from build123d import *

# Parameters (mm, degrees)
GAP_DEPTH               = 39.247748954
CUT_EXTRUDE1_DEPTH      = 6.35
CUT_EXTRUDE1_DEPTH_BACK = 6.35
SKETCH3_R               = 4.928370377
SKETCH3_R_2             = 2.3495


with BuildPart() as part:
    # Sketch1 → Base-Revolve (revolve)
    with BuildSketch(Plane.XY, mode=Mode.PRIVATE) as base_revolve_sk:
        Polygon((0, 1.3589), (38.1, 1.3589), (38.1, 2.159), (36.703, 2.3749), (1.397, 2.3749), (0, 2.159), align=None)
    revolve(base_revolve_sk.sketch.rotate(Axis((-9.525, 0, 0), (1, 0, 0)), 90), axis=Axis((-9.525, 0, 0), (1, 0, 0)))

    # Sketch2 → Gap (cut, through all)
    with BuildSketch(Plane(origin=(0, 0, 0), x_dir=(0, -1, 0), z_dir=(-1, 0, 0))):
        with BuildLine():
            Line((0, 0), (0.190059157, 2.414930555))
            ThreePointArc((0.190059157, 2.414930555), (0, 2.422398), (-0.190059157, 2.414930555))
            Line((-0.190059157, 2.414930555), (0, 0))
        make_face()
    extrude(amount=-GAP_DEPTH, mode=Mode.SUBTRACT)

    # Sketch3 → Cut-Extrude1 (cut, two sides: drawn at the far end of the back side and taken through both)
    with BuildSketch(Plane(origin=(17.78, 0, 0), x_dir=(0, 0, -1), z_dir=(1, 0, 0)).offset(-CUT_EXTRUDE1_DEPTH_BACK)):
        Circle(SKETCH3_R)
        Circle(SKETCH3_R_2, mode=Mode.SUBTRACT)
    extrude(amount=CUT_EXTRUDE1_DEPTH + CUT_EXTRUDE1_DEPTH_BACK, mode=Mode.SUBTRACT)


solid = part.part
Source: CAD feature listing. Evaluate the final solid. Frame: model axes, mm. A direction names the side the tool comes from. Coordinates: 2 decimals unless noted, no trailing zeros. Write each loop counter-clockwise with the first axis right and the second up, starting at its lowest first coordinate (ties: lowest second). Pieces come first, ordered by that corner, then holes. Notation, with made-up numbers: M -30,62.5 L 5,62.5 A13 ccw 5,79.5 Z; hole C 59.25,-28 d11. An arc over 180 degrees is marked long. Use a Markdown table: item, result.
1) Section B-B, the plane x = 3. Output: boundary loops of the cut face in (y, z), then the cut area to 3 significant figures.
Conclusion:
| item | result |
|---|---|
| outline | M -0.19,2.37 A2.37 ccw long 0.19,2.37 L 0.11,1.35 A1.36 cw long -0.11,1.35 Z |
| area | 11.6 mm^2 |
2) Mould query, pull axis Z, two halves, no side actions, for faces 3 (the flat face through (18.783, 0.147, 1.868)), 4 (the conical face through (0.378, -0.095, -2.215)), 5 (the cylindrical face through (19.317, -0.058, -1.358)). Classes: pulls with the +Z half, pulls with the -Z half, needs draft (parallel to the pull), parting line crosses it, or undercut.
Conclusion:
| item | result |
|---|---|
| face 3 | pulls with the +Z half |
| face 4 | parting line crosses it |
| face 5 | undercut |
3) First-contact query: pin 1 Ø2 at (y, z) = (-1.5, -0.5) entering from -X; pin 2 Ø2 at (x, y) = (20.5, 0) entering from -Z. Flat tips, straight axial feed; report the tip coordinate or a pass-through.
Conclusion:
| item | result |
|---|---|
| pin 1 | stops at x = 0 |
| pin 2 | stops at z = -2.35 |
4) Ray query, L1, parallel to Y at x = 21, z = 0; L2, parallel to Y at x = 28.5, z = 0; L3, parallel to Z at x = 19, y = 0. Return the intervals inside material, ascending.
Conclusion:
| item | result |
|---|---|
| L1 | y = -2.35 to -1.36, 1.36 to 2.35 |
| L2 | y = -2.37 to -1.36, 1.36 to 2.37 |
| L3 | z = -2.35 to -1.36 |
5) Reachability of faces 1 (the flat face through (18.783, -0.146, 1.854)), 2 (the conical face through (37.7, -0.1, -2.22)) from +Z, -Z, +X, -X, +Y, -Y: full face, straight path, thin tool, end or side. Return the list, or none.
Conclusion:
| item | result |
|---|---|
| face 1 | +Z, +X, -X |
| face 2 | +X |
